The listing builds one solid part. Answer for the finished solid, in the listing's coordinates (mm). Face numbers are marked on the shaded views. A direction names the side the tool comes from. Coordinates: 2 decimals unless noted, no trailing zeros. Loops run counter-clockwise (first coordinate to the right, second up) from the corner with the lowest first, then second, coordinate; pieces in that order, holes last. Notation, with made-up numbers: (83, 25) -> (101, 25) arc R24 cw to (101, 43) -> close; hole circle Ø11 at (58, -22.75). An arc over 180 degrees is marked (long way). Answer in a Markdown table with one row per item.
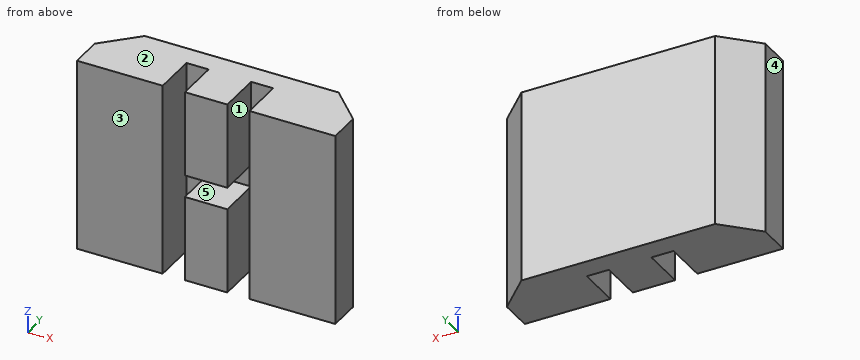
```python
from build123d import *

# Parameters (mm, degrees)
SKETCH2_W             = 39.85
SKETCH2_H             = 90
BOSS_EXTRUDE1_DEPTH   = 20
BOSS_EXTRUDE1_2_DEPTH = 20
BOSS_EXTRUDE1_3_DEPTH = 20
BOSS_EXTRUDE1_4_DEPTH = 20
SKETCH3_W             = 120
SKETCH3_H             = 90
BOSS_EXTRUDE2_DEPTH   = 10
CUT_EXTRUDE2_DEPTH    = 114


with BuildPart() as part:
    # Sketch2 → Boss-Extrude1 (new body)
    with BuildSketch(Plane(origin=(0, 0, 0), x_dir=(1, 0, 0), z_dir=(0, 1, 0))):
        with Locations((-0.075, 90)):
            Rectangle(SKETCH2_W, SKETCH2_H)
    extrude(amount=BOSS_EXTRUDE1_DEPTH)



with BuildPart() as body_2:
    # Sketch2 → Boss-Extrude1 2 (new body)
    with BuildSketch(Plane(origin=(0, 0, 0), x_dir=(1, 0, 0), z_dir=(0, 1, 0))):
        Polygon((49.85, 95.15), (49.85, 134.85), (49.85, 135), (30.15, 135), (30.15, 134.85), (30.15, 95.15), align=None)
    extrude(amount=BOSS_EXTRUDE1_2_DEPTH)


with BuildPart() as body_3:
    # Sketch2 → Boss-Extrude1 3 (new body)
    with BuildSketch(Plane(origin=(0, 0, 0), x_dir=(1, 0, 0), z_dir=(0, 1, 0))):
        Polygon((49.85, 45.15), (49.85, 45), (30.15, 45), (30.15, 45.15), (30.15, 84.85), (49.85, 84.85), align=None)
    extrude(amount=BOSS_EXTRUDE1_3_DEPTH)


with BuildPart() as body_4:
    # Sketch2 → Boss-Extrude1 4 (new body)
    with BuildSketch(Plane(origin=(0, 0, 0), x_dir=(1, 0, 0), z_dir=(0, 1, 0))):
        with Locations((80.075, 90)):
            Rectangle(SKETCH2_W, SKETCH2_H)
    extrude(amount=BOSS_EXTRUDE1_4_DEPTH)


with BuildPart() as part_1:
    add(part.part)

    add(body_2.part)  # Boss-Extrude2 merges body 2

    add(body_3.part)  # Boss-Extrude2 merges body 3

    add(body_4.part)  # Boss-Extrude2 merges body 4
    # Sketch3 → Boss-Extrude2 (add)
    with BuildSketch(Plane(origin=(0, 20, 0), x_dir=(1, 0, 0), z_dir=(0, 1, 0))):
        with Locations((40, 90)):
            Rectangle(SKETCH3_W, SKETCH3_H)
    extrude(amount=BOSS_EXTRUDE2_DEPTH)

    # Sketch5 → Cut-Extrude2 (cut)
    with BuildSketch(Plane.XY.offset(-45)):
        Polygon((-20, 30), (-20, 15), (-5, 30), align=None)
        Polygon((100, 30), (85, 30), (100, 15), align=None)
    extrude(amount=-CUT_EXTRUDE2_DEPTH, mode=Mode.SUBTRACT)


solid = part_1.part
```
Item 1: A cutting plane is placed at B-B, the plane x = 37.5. Determine the outline of the cut face in (y, z), plus the area to 3 significant figures.
Findings below:
| item | result |
|---|---|
| outline | (0, -135) -> (30, -135) -> (30, -45) -> (0, -45) -> (0, -84.85) -> (20, -84.85) -> (20, -95.15) -> (0, -95.15) -> close |
| area | 2,490 mm2 |
Item 2: A flat-ended cylindrical pin translates along its axis: pin 1 Ø2 at (x, y) = (50.5, 8.5) entering from +Z. Find the tip coordinate at first contact, or state that the pin passes through.
Findings below:
| item | result |
|---|---|
| pin 1 | stops at z = -45 |
Item 3: A cutting plane is placed at C-C, the plane y = 25.75. Determine the outline of the cut face in (x, z).
Findings below:
| item | result |
|---|---|
| outline | (-9.25, -135) -> (89.25, -135) -> (89.25, -45) -> (-9.25, -45) -> close |
Item 4: A cutting plane is placed at A-A, the plane z = -111. Determine the outline of the cut face in (x, y).
Findings below:
| item | result |
|---|---|
| outline | (-20, 0) -> (19.85, 0) -> (19.85, 20) -> (30.15, 20) -> (30.15, 0) -> (49.85, 0) -> (49.85, 20) -> (60.15, 20) -> (60.15, 0) -> (100, 0) -> (100, 15) -> (85, 30) -> (-5, 30) -> (-20, 15) -> close |
Item 5: A cutting plane is placed at D-D, the plane x = -7. Determine the outline of the cut face in (y, z).
Findings below:
| item | result |
|---|---|
| outline | (0, -135) -> (28, -135) -> (28, -45) -> (0, -45) -> close |
Item 6: Find the intervals of material crossed by probe 1 along X at (y, z) = (7, -115.5); probe 2 along X at (y, z) = (16.25, -116); probe 3 along Y at (x, z) = (95, -113), in increasing order.
Findings below:
| item | result |
|---|---|
| probe 1 | x = -20 to 19.85, 30.15 to 49.85, 60.15 to 100 |
| probe 2 | x = -18.75 to 19.85, 30.15 to 49.85, 60.15 to 98.75 |
| probe 3 | y = 0 to 20 |
Item 7: A tool of negligible diameter and unlimited length cuts with its end or side. For the marked faces 1 and 2, from which of +Z, -Z, +X, -X, +Y, -Y can it reach the whole face along a straight path? Write none if from no direction.
Findings below:
| item | result |
|---|---|
| face 1 | +Z, -Z, -Y |
| face 2 | +Z, +X, -X, +Y, -Y |
Item 8: Determine the mould class of the marked faces 3, 4 and 5 for opening direction X: +X half, -X half, draft (parallel to the pull), parting line (faces both ways), or undercut.
Findings below:
| item | result |
|---|---|
| face 3 | draft |
| face 4 | -X half |
| face 5 | undercut |
